from build123d import *

# Parameters (mm, degrees)
BOSS_EXTRUDE1_DEPTH = 12
CUT_EXTRUDE1_DEPTH  = 2
SKETCH3_R           = 2.5
SKETCH3_R_2         = 1.5
BOSS_EXTRUDE2_DEPTH = 1.2
SKETCH4_R           = 2.5
BOSS_EXTRUDE3_DEPTH = 5
CHAMFER1_SIZE       = 0.5
SKETCH5_R           = 1.5
CUT_EXTRUDE2_DEPTH  = 5


with BuildPart() as part:
    # Sketch1 → Boss-Extrude1 (new body)
    with BuildSketch(Plane(origin=(0, 0, 0), x_dir=(1, 0, 0), z_dir=(0, 1, 0))):
        with BuildLine():
            Line((-23.25, -5), (-5.749755012, -5))
            Line((-5.749755012, -5), (-5.749755012, 0))
            add(Edge.make_bspline(
                [(-3.25, 5), (-5.749755012, 5), (-5.749755012, 0)],
                knots=[0, 0, 0, 1.570796327, 1.570796327, 1.570796327], degree=2, weights=[1, 0.707106781, 1]))
            Line((-3.25, 5), (3.25, 5))
            add(Edge.make_bspline(
                [(5.748694825, 0), (5.748694825, 5), (3.25, 5)],
                knots=[4.71238898, 4.71238898, 4.71238898, 6.283185307, 6.283185307, 6.283185307], degree=2, weights=[1, 0.707106781, 1]))
            Line((5.748694825, 0), (5.748694825, -5))
            Line((5.748694825, -5), (23.25, -5))
            Line((23.25, -5), (23.25, -3))
            Line((23.25, -3), (23.25, -1))
            Line((23.25, -1), (9.3, -1))
            ThreePointArc((9.3, -1), (8.592893219, -0.707106781), (8.3, 0))
            Line((8.3, 0), (8.3, 6.6))
            Line((8.3, 6.6), (-8.3, 6.6))
            Line((-8.3, 6.6), (-8.3, 0))
            ThreePointArc((-8.3, 0), (-8.592893219, -0.707106781), (-9.3, -1))
            Line((-9.3, -1), (-23.25, -1))
            Line((-23.25, -1), (-23.25, -5))
        make_face()
    extrude(amount=BOSS_EXTRUDE1_DEPTH)

    # Sketch2 → Cut-Extrude1 (cut)
    with BuildSketch(Plane(origin=(0, 0, 1), x_dir=(-1, 0, 0), z_dir=(0, 0, -1))):
        Polygon((19.85850269, 6), (18.068716856, 9.1), (14.489145187, 9.1), (12.699359352, 6), (14.489145187, 2.9), (18.068716856, 2.9), align=None)
        Polygon((-12.686507152, 6), (-14.476292987, 9.1), (-18.055864656, 9.1), (-19.84565049, 6), (-18.055864656, 2.9), (-14.476292987, 2.9), align=None)
    extrude(amount=-CUT_EXTRUDE1_DEPTH, mode=Mode.SUBTRACT)

    # Sketch3 → Boss-Extrude2 (add)
    with BuildSketch(Plane(origin=(0, 12, 0), x_dir=(1, 0, 0), z_dir=(0, 1, 0))):
        with BuildLine():
            Line((-8.3, 6.6), (8.3, 6.6))
            Line((8.3, 6.6), (8.3, 10.6))
            ThreePointArc((8.3, 10.6), (0, 13.462912018), (-8.3, 10.6))
            Line((-8.3, 10.6), (-8.3, 6.6))
        make_face()
        with Locations(Location((-3.25, 9.48526903, 0), (0, 0, 270))):
            Circle(SKETCH3_R, mode=Mode.SUBTRACT)
        with Locations(Location((3.25, 9.48526903, 0), (0, 0, 270))):
            Circle(SKETCH3_R_2, mode=Mode.SUBTRACT)
    extrude(amount=-BOSS_EXTRUDE2_DEPTH)

    # Sketch4 → Boss-Extrude3 (add)
    with BuildSketch(Plane.XZ.offset(-10.8)):
        with BuildLine():
            Line((8.3, -6.6), (-8.3, -6.6))
            Line((-8.3, -6.6), (-8.3, -10.6))
            ThreePointArc((-8.3, -10.6), (0, -13.462912018), (8.3, -10.6))
            Line((8.3, -10.6), (8.3, -6.6))
        make_face()
        with Locations(Location((-3.25, -9.48526903, 0), (0, 0, 90))):
            Circle(SKETCH4_R, mode=Mode.SUBTRACT)
        with Locations(Location((3.25, -9.48526903, 0), (0, 0, 270))):
            Circle(SKETCH4_R, mode=Mode.SUBTRACT)
    extrude(amount=BOSS_EXTRUDE3_DEPTH)

    # Chamfer1
    chamfer1_edges = [part.edges().sort_by_distance(p)[0] for p in [
        (0, 12, -5),
        (-5.260112096, 12, -2.972310439),
        (5.259369228, 12, -2.972013605),
        (-5.749755012, 12, 2.5),
        (5.748694825, 12, 2.5),
    ]]
    chamfer(chamfer1_edges, length=CHAMFER1_SIZE)

    # Sketch5 → Cut-Extrude2 (cut)
    with BuildSketch(Plane(origin=(0, 0, 1), x_dir=(-1, 0, 0), z_dir=(0, 0, -1))):
        with Locations((-16.266078821, 6)):
            Circle(SKETCH5_R)
        with Locations((16.278931021, 6)):
            Circle(SKETCH5_R)
    extrude(amount=-CUT_EXTRUDE2_DEPTH, mode=Mode.SUBTRACT)


solid = part.part
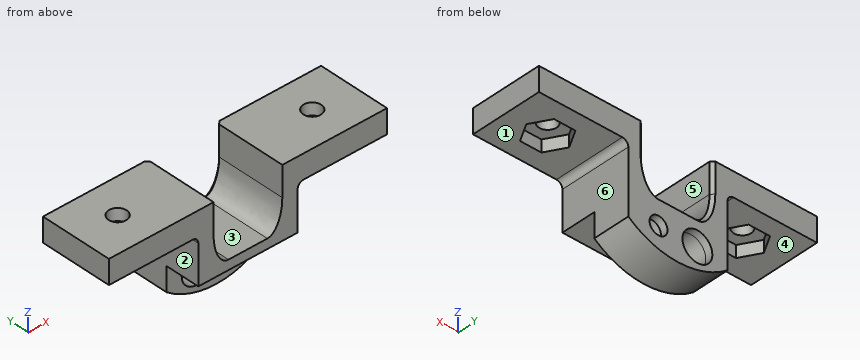
The model under review builds one solid part; all positions refer to its coordinate system, in mm. Face numbers are marked on the shaded views. A direction names the side the tool comes from. Give positions to 0.01 mm unless a question says otherwise; leave off trailing zeros. Write each loop counter-clockwise with the first axis right and the second up, starting at its lowest first coordinate (ties: lowest second). Pieces come first, ordered by that corner, then holes.
1. Wall thickness on L1, parallel to X at y = 9.25, z = 4; L2, parallel to X at y = 4.5, z = 1.25; L3, parallel to Z at x = -2.5, y = 5.75: over which ranges is each line inside the solid? List them lowest first.
2. Add section D-D, the plane z = -10. Write out the cut boundary in (x, y), plus the area to 3 significant figures.
3. Draft analysis for pull direction X (two halves, no side actions). For the marked faces 4, 5 and 6, state which applies: +X half, -X half, draft (parallel to the pull), parting line (faces both ways), or undercut.
4. Tool access review of the marked faces 1, 2 and 3: name each direction out of +Z, -Z, +X, -X, +Y, -Y from which nothing blocks a thin tool from reaching the whole face with its end or side.
5. Add section A-A, the plane z = 3.5. Write out the cut boundary in (x, y).
6. For P1, Ø1.8, axis at x = 16.27, y = 6, coming from the +Z side; P2, Ø4, axis at x = 8.5, y = 6.5, coming from the -Z side; P3, Ø2.5, axis at x = 3.5, z = -10, coming from the -Y side; P4, Ø6, axis at x = -18.5, y = 6, coming from the -Z side, all flat-tipped, find the tip position at first contact; note any pin that passes through.
7. Add section B-B, the plane x = -16. Write out the cut boundary in (y, z), plus the area to 3 significant figures.
8. Add section C-C, the plane z = 1.5. Write out the cut boundary in (x, y), plus the area to 3 significant figures.
Worked answers:
1. L1: x = -23.25 to -5.75, 5.75 to 23.25
1. L2: x = -23.25 to -18.99, -13.57 to -5.75, 5.75 to 13.55, 18.98 to 23.25
1. L3: z = -6.6 to -5
2. outline: (-8.3, 5.8) - (-5.7, 5.8) - (-5.7, 12) - (-8.3, 12) - close; (-0.8, 5.8) - (0.8, 5.8) - (0.8, 10.8) - (1.84, 10.8) - (1.84, 12) - (-0.8, 12) - close; (4.66, 10.8) - (5.7, 10.8) - (5.7, 5.8) - (8.3, 5.8) - (8.3, 12) - (4.66, 12) - close
2. area: 44.7 mm2
3. face 4: draft
3. face 5: undercut
3. face 6: +X half
4. face 1: -Z, +X, +Y, -Y
4. face 2: -Z, -X, +Y, -Y
4. face 3: +Z, +Y, -Y
5. outline: (-23.25, 0) - (-5.75, 0) - (-5.75, 11.5) - (-6.25, 12) - (-23.25, 12) - close; (5.75, 0) - (23.25, 0) - (23.25, 12) - (6.25, 12) - (5.75, 11.5) - close; hole circle Ø3 at (-16.28, 6); hole circle Ø3 at (16.27, 6)
6. P1: passes through
6. P2: stops at z = -11.79
6. P3: stops at y = 10.8
6. P4: stops at z = 1
7. outline: (0, 1) - (2.9, 1) - (2.9, 3) - (4.53, 3) - (4.53, 5) - (0, 5) - close; (7.47, 3) - (9.1, 3) - (9.1, 1) - (12, 1) - (12, 5) - (7.47, 5) - close
7. area: 29.7 mm2
8. outline: (-23.25, 0) - (-5.75, 0) - (-5.75, 11.5) - (-6.25, 12) - (-23.25, 12) - close; (5.75, 0) - (23.25, 0) - (23.25, 12) - (6.25, 12) - (5.75, 11.5) - close; hole (-19.86, 6) - (-18.07, 2.9) - (-14.49, 2.9) - (-12.7, 6) - (-14.49, 9.1) - (-18.07, 9.1) - close; hole (12.69, 6) - (14.48, 2.9) - (18.06, 2.9) - (19.85, 6) - (18.06, 9.1) - (14.48, 9.1) - close
8. area: 353 mm2
